```python
from build123d import *

# Parameters (mm, degrees)
ESQUISSE1_R              = 7.5
ESQUISSE1_R_2            = 2.3
BOSS_EXTRU_1_DEPTH       = 6
ENL_V_MAT_EXTRU_9_DEPTH  = 10.5
ESQUISSE6_R              = 2.3
ENL_V_MAT_EXTRU_10_DEPTH = 50
ENL_V_MAT_EXTRU_11_DEPTH = 50
ESQUISSE9_R              = 2.5
ENL_V_MAT_EXTRU_12_DEPTH = 35
ESQUISSE3_R              = 2.3
ENL_V_MAT_EXTRU_13_DEPTH = 35
ESQUISSE10_R             = 2.3
ENL_V_MAT_EXTRU_14_DEPTH = 10


with BuildPart() as part:
    # Esquisse1 → Boss.-Extru.1 (new body)
    with BuildSketch(Plane(origin=(0, 0, 0), x_dir=(1, 0, 0), z_dir=(0, 1, 0))):
        Polygon((-150, 0), (-150, 260), (-110, 300), (110, 300), (150, 260), (150, 0), align=None)
        with Locations(Location((-120, 30, 0), (0, 0, 270))):
            Circle(ESQUISSE1_R, mode=Mode.SUBTRACT)
        with Locations(Location((-120, 267.5, 0), (0, 0, 270))):
            Circle(ESQUISSE1_R, mode=Mode.SUBTRACT)
        with Locations(Location((120, 268.5, 0), (0, 0, 270))):
            Circle(ESQUISSE1_R, mode=Mode.SUBTRACT)
        with Locations(Location((-111.514718626, 275.985281374, 0), (0, 0, 270))):
            Circle(ESQUISSE1_R_2, mode=Mode.SUBTRACT)
        with Locations(Location((-128.485281374, 259.014718626, 0), (0, 0, 270))):
            Circle(ESQUISSE1_R_2, mode=Mode.SUBTRACT)
        with Locations(Location((111.514718626, 276.985281374, 0), (0, 0, 270))):
            Circle(ESQUISSE1_R_2, mode=Mode.SUBTRACT)
        with Locations(Location((128.485281374, 260.014718626, 0), (0, 0, 270))):
            Circle(ESQUISSE1_R_2, mode=Mode.SUBTRACT)
        with Locations(Location((120, 30, 0), (0, 0, 270))):
            Circle(ESQUISSE1_R, mode=Mode.SUBTRACT)
        with Locations(Location((120, 42, 0), (0, 0, 270))):
            Circle(ESQUISSE1_R_2, mode=Mode.SUBTRACT)
        with Locations(Location((-120, 42, 0), (0, 0, 270))):
            Circle(ESQUISSE1_R_2, mode=Mode.SUBTRACT)
        with Locations(Location((-120, 18, 0), (0, 0, 270))):
            Circle(ESQUISSE1_R_2, mode=Mode.SUBTRACT)
        with Locations(Location((-132, 30, 0), (0, 0, 270))):
            Circle(ESQUISSE1_R_2, mode=Mode.SUBTRACT)
        with Locations(Location((-108, 30, 0), (0, 0, 270))):
            Circle(ESQUISSE1_R_2, mode=Mode.SUBTRACT)
        with Locations(Location((108, 30, 0), (0, 0, 270))):
            Circle(ESQUISSE1_R_2, mode=Mode.SUBTRACT)
        with Locations(Location((132, 30, 0), (0, 0, 270))):
            Circle(ESQUISSE1_R_2, mode=Mode.SUBTRACT)
        with Locations(Location((120, 18, 0), (0, 0, 270))):
            Circle(ESQUISSE1_R_2, mode=Mode.SUBTRACT)
    extrude(amount=BOSS_EXTRU_1_DEPTH)

    # Esquisse7 → Enlèv. mat.-Extru.9 (cut)
    with BuildSketch(Plane(origin=(0, 6, 0), x_dir=(1, 0, 0), z_dir=(0, 1, 0))):
        Polygon((-130, 150), (-130, 182), (-140, 182), (-140, 118), (-130, 118), align=None)
    enl_v_mat_extru_9 = extrude(amount=-ENL_V_MAT_EXTRU_9_DEPTH, mode=Mode.SUBTRACT)

    # Esquisse6 → Enlèv. mat.-Extru.10 (cut)
    with BuildSketch(Plane(origin=(0, 6, 0), x_dir=(1, 0, 0), z_dir=(0, 1, 0))):
        with Locations(Location((110, 210, 0), (0, 0, 270))):
            Circle(ESQUISSE6_R)
        with Locations(Location((138.5, 210, 0), (0, 0, 270))):
            Circle(ESQUISSE6_R)
        with Locations(Location((138.5, 188, 0), (0, 0, 270))):
            Circle(ESQUISSE6_R)
        with Locations(Location((110, 188, 0), (0, 0, 270))):
            Circle(ESQUISSE6_R)
        with Locations(Location((-138.5, 90, 0), (0, 0, 270))):
            Circle(ESQUISSE6_R)
        with Locations(Location((-138.5, 112, 0), (0, 0, 270))):
            Circle(ESQUISSE6_R)
        with Locations(Location((-110, 112, 0), (0, 0, 270))):
            Circle(ESQUISSE6_R)
        with Locations(Location((-110, 90, 0), (0, 0, 270))):
            Circle(ESQUISSE6_R)
    enl_v_mat_extru_10 = extrude(amount=-ENL_V_MAT_EXTRU_10_DEPTH, mode=Mode.SUBTRACT)

    # Esquisse4 → Enlèv. mat.-Extru.11 (cut)
    with BuildSketch(Plane(origin=(0, 6, 0), x_dir=(1, 0, 0), z_dir=(0, 1, 0))):
        Polygon((-100, 150), (-100, 182), (-64, 182), (-64, 118), (-100, 118), align=None)
    enl_v_mat_extru_11 = extrude(amount=-ENL_V_MAT_EXTRU_11_DEPTH, mode=Mode.SUBTRACT)

    # Symétrie1: Enlèv. mat.-Extru.9 across plane
    add(enl_v_mat_extru_9.mirror(Plane(origin=(0, 0, 0), x_dir=(0, 0, 1), z_dir=(1, 0, 0))), mode=Mode.SUBTRACT)

    # Symétrie2: Enlèv. mat.-Extru.11 across plane
    add(enl_v_mat_extru_11.mirror(Plane(origin=(0, 0, 0), x_dir=(0, 0, 1), z_dir=(1, 0, 0))), mode=Mode.SUBTRACT)

    # Symétrie3: Enlèv. mat.-Extru.10 across plane
    add(enl_v_mat_extru_10.mirror(Plane(origin=(0, 0, 0), x_dir=(0, 0, 1), z_dir=(1, 0, 0))), mode=Mode.SUBTRACT)

    # Esquisse9 → Enlèv. mat.-Extru.12 (cut)
    with BuildSketch(Plane(origin=(0, 6, 0), x_dir=(1, 0, 0), z_dir=(0, 1, 0))):
        with Locations(Location((-100, 50, 0), (0, 0, 270))):
            Circle(ESQUISSE9_R)
        with Locations(Location((100, 50, 0), (0, 0, 270))):
            Circle(ESQUISSE9_R)
        with Locations(Location((100, 250, 0), (0, 0, 270))):
            Circle(ESQUISSE9_R)
        with Locations(Location((-100, 250, 0), (0, 0, 270))):
            Circle(ESQUISSE9_R)
    extrude(amount=-ENL_V_MAT_EXTRU_12_DEPTH, mode=Mode.SUBTRACT)

    # Esquisse3 → Enlèv. mat.-Extru.13 (cut)
    with BuildSketch(Plane(origin=(0, 6, 0), x_dir=(1, 0, 0), z_dir=(0, 1, 0))):
        with Locations(Location((-60, 174, 0), (0, 0, 270))):
            Circle(ESQUISSE3_R)
        with Locations(Location((-60, 116, 0), (0, 0, 270))):
            Circle(ESQUISSE3_R)
        with Locations(Location((-30, 166, 0), (0, 0, 270))):
            Circle(ESQUISSE3_R)
        with Locations(Location((-30, 124, 0), (0, 0, 270))):
            Circle(ESQUISSE3_R)
        with Locations(Location((60, 184, 0), (0, 0, 270))):
            Circle(ESQUISSE3_R)
        with Locations(Location((30, 176, 0), (0, 0, 270))):
            Circle(ESQUISSE3_R)
        with Locations(Location((30, 134, 0), (0, 0, 270))):
            Circle(ESQUISSE3_R)
        with Locations(Location((60, 126, 0), (0, 0, 270))):
            Circle(ESQUISSE3_R)
    extrude(amount=-ENL_V_MAT_EXTRU_13_DEPTH, mode=Mode.SUBTRACT)

    # Esquisse10 → Enlèv. mat.-Extru.14 (cut)
    with BuildSketch(Plane(origin=(0, 6, 0), x_dir=(1, 0, 0), z_dir=(0, 1, 0))):
        with Locations(Location((-33, 227, 0), (0, 0, 270))):
            Circle(ESQUISSE10_R)
        with Locations(Location((-19, 73, 0), (0, 0, 270))):
            Circle(ESQUISSE10_R)
        with Locations(Location((33, 73, 0), (0, 0, 270))):
            Circle(ESQUISSE10_R)
        with Locations(Location((-33, 183, 0), (0, 0, 270))):
            Circle(ESQUISSE10_R)
        with Locations(Location((33, 117, 0), (0, 0, 270))):
            Circle(ESQUISSE10_R)
        with Locations(Location((-19, 117, 0), (0, 0, 270))):
            Circle(ESQUISSE10_R)
        with Locations(Location((19.4, 227, 0), (0, 0, 270))):
            Circle(ESQUISSE10_R)
        with Locations(Location((19.4, 183, 0), (0, 0, 270))):
            Circle(ESQUISSE10_R)
    extrude(amount=-ENL_V_MAT_EXTRU_14_DEPTH, mode=Mode.SUBTRACT)


solid = part.part
```
For this review, take the finished solid that the model builds, in its own axes (mm). Round coordinates to 2 decimals unless told otherwise and drop trailing zeros. Write each loop counter-clockwise with the first axis right and the second up, starting at its lowest first coordinate (ties: lowest second). Pieces come first, ordered by that corner, then holes. Notation, with made-up numbers: (-15.75, 32.25) -> (31.25, 32.25) arc R25 cw to (31.25, 66.25) -> close; hole circle Ø7 at (37, 39). An arc over 180 degrees is marked (long way). Use one line per item in the form item = value.
Q1. To check wall thickness, follow probe 1 along X at (y, z) = (2.5, -157.5); probe 2 along X at (y, z) = (0.7, -166); probe 3 along X at (y, z) = (4.45, -188). State the ranges of each line that lie inside material, in increasing order. Write a range as from..to.
Resolved:
probe_1 = -150..-140, -130..-100, -64..64, 100..130, 140..150
probe_2 = -150..-140, -130..-100, -64..-32.3, -27.7..64, 100..130, 140..150
probe_3 = -150..-140.8, -136.2..-112.3, -107.7..107.7, 112.3..136.2, 140.8..150
Q2. Clearance check with flat-ended pins moving along their axes: pin 1 Ø3 at (x, z) = (110, -188) entering from -Y; pin 2 Ø3 at (x, y) = (-136.5, 1.5) entering from -Z. State where each tip first meets the part, or that it passes through.
Resolved:
pin_1 = through
pin_2 = -275
Q3. Consider section B-B (x = 93). State the section outline as (y, z) points.
Resolved:
outline = (0, -300) -> (6, -300) -> (6, -182) -> (0, -182) -> close; (0, -118) -> (6, -118) -> (6, 0) -> (0, 0) -> close
Q4. The part is to be moulded in two halves that separate along Z. For faces 1 (the flat face through (-130, 3, -280)), 2 (the flat face through (2, 6, -152)), 3 (the cylindrical face through (117.13, 2.96, -261.57)), say which applies: released by +Z, released by -Z, zero draft, split by the parting line, or undercut.
Resolved:
face_1 = released by -Z
face_2 = zero draft
face_3 = undercut
Q5. Consider section C-C (y = 5.1). State how many separate pieces and enclosed holes the cut face has, then the cut area to 3 significant figures.
Resolved:
separate_pieces = 1
enclosed_holes = 56
area = 81,000 mm²
Q6. Consider section A-A (z = -143.5). State the section outline as (x, y) points.
Resolved:
outline = (-150, 0) -> (-140, 0) -> (-140, 6) -> (-150, 6) -> close; (-130, 0) -> (-100, 0) -> (-100, 6) -> (-130, 6) -> close; (-64, 0) -> (64, 0) -> (64, 6) -> (-64, 6) -> close; (100, 0) -> (130, 0) -> (130, 6) -> (100, 6) -> close; (140, 0) -> (150, 0) -> (150, 6) -> (140, 6) -> close
